Verification items for the finished model (mm, model axes). A direction names the side the tool comes from. Give positions to 0.01 mm unless a question says otherwise; leave off trailing zeros. Loops run counter-clockwise (first coordinate to the right, second up) from the corner with the lowest first, then second, coordinate; pieces in that order, holes last. Notation, with made-up numbers: M 54,75.5 L 61,75.5 A18 ccw 61,100.5 Z; hole C 27,-39 d4. An arc over 180 degrees is marked long. Use CSV: the item, a comma, the result in double quotes.
Solid Edge part; units mm, degrees
sketch "Sketch1" plane through (0, 0, 0) normal (1, 0, 0) x (0, 1, 0)
  circle A0 centre (0, 0) radius 14
extrude "Protrusion1" add sketch "Sketch1" along normal mid plane 450
sketch "Sketch2" plane through (225, 0, 0) normal (1, 0, 0) x (0, 1, 0)
  line L0 (-26, 0) -> (-26, 32)
  line L1 (-26, 32) -> (26, 32)
  line L2 (26, 32) -> (26, 0)
  arc A0 (-26, 0) -> (26, 0) centre (0, 0) ccw
extrude "Protrusion2" add sketch "Sketch2" along normal blind 10
mirror "Mirror1" about plane through (0, 0, 0) normal (1, 0, 0) of "Protrusion2"
(1) Scan lines: L1, parallel to X at y = 12, z = 13; L2, parallel to Y at x = 186, z = 0.5; L3, parallel to Z at x = -28.5, y = 1. Record each from-to range of solid material in increasing order. Write a range as from..to.
Calculated:
L1,"x = -235..-225, 225..235"
L2,"y = -13.99..13.99"
L3,"z = -13.96..13.96"
(2) Depth check by flat-ended pin: pin 1 Ø3 at (x, z) = (84, -16.5) entering from +Y; pin 2 Ø10 at (x, z) = (-8, -1.5) entering from +Y; pin 3 Ø8 at (x, y) = (116.5, -14) entering from +Z; pin 4 Ø5 at (x, y) = (46.5, -14) entering from +Z. Enter the tip coordinate at first touch or a pass-through.
Calculated:
pin 1,"passes through"
pin 2,"stops at y = 14"
pin 3,"stops at z = 9.8"
pin 4,"stops at z = 7.98"
(3) Section check B-B on y = 18. Record the cut outline in (x, z), plus the area to 3 significant figures.
Calculated:
outline,"M -235,-18.76 L -225,-18.76 L -225,32 L -235,32 Z; M 225,-18.76 L 235,-18.76 L 235,32 L 225,32 Z"
area,"1,020 mm²"
(4) Section check A-A on z = -19.5. Record the cut outline in (x, y), plus the area to 3 significant figures.
Calculated:
outline,"M -235,-17.2 L -225,-17.2 L -225,17.2 L -235,17.2 Z; M 225,-17.2 L 235,-17.2 L 235,17.2 L 225,17.2 Z"
area,"688 mm²"
(5) Section check C-C on x = -186.5. Record the cut outline in (y, z).
Calculated:
outline,"C 0,0 d28"
(6) Tool access check on faces 4 (the cylindrical face through (3.15, 12.932, -5.362)), 5 (the flat face through (-230, 0, 32)). Record the directions out of +Z, -Z, +X, -X, +Y, -Y that give a thin tool (end or side, any length) a straight path to the whole face; none if there is none.
Calculated:
face 4,"none"
face 5,"+Z, +X, -X, +Y, -Y"
(7) Mould release check, pull along X, two halves, no side actions. Record for faces 1 (the flat face through (230, 26, 16)), 2 (the flat face through (-225, 0, 15)), 3 (the flat face through (235, 0, 3)): released by +X, released by -X, zero draft, split by the parting line, or undercut.
Calculated:
face 1,"zero draft"
face 2,"undercut"
face 3,"released by +X"
